```python
from build123d import *

# Parameters (mm, degrees)
SKETCH_2_R      = 3
SKETCH_2_R_2    = 1
EXTRUDE_1_DEPTH = 6
EXTRUDE_2_DEPTH = 5
SKETCH_6_R      = 3
SKETCH_6_R_2    = 1
EXTRUDE_3_DEPTH = 6
FILLET_1_R      = 1


with BuildPart() as part:
    # Эскиз2 → Бобышка-Вытянуть1 (new, symmetric)
    with BuildSketch(Plane.XY):
        Circle(SKETCH_2_R)
        Circle(SKETCH_2_R_2, mode=Mode.SUBTRACT)
    extrude(amount=EXTRUDE_1_DEPTH, both=True)

    # Эскиз4 → Бобышка-Вытянуть2 (add, symmetric)
    with BuildSketch(Plane.XY):
        with BuildLine():
            Line((2.236067977, 2), (23, 2))
            Line((23, 2), (23, -2))
            Line((23, -2), (2.236067977, -2))
            ThreePointArc((2.236067977, -2), (3, 0), (2.236067977, 2))
        make_face()
    extrude(amount=EXTRUDE_2_DEPTH, both=True)

    # Эскиз6 → Бобышка-Вытянуть3 (add, symmetric)
    with BuildSketch(Plane.XY):
        with Locations((24, 0)):
            Circle(SKETCH_6_R)
        with Locations((24, 0)):
            Circle(SKETCH_6_R_2, mode=Mode.SUBTRACT)
    extrude(amount=EXTRUDE_3_DEPTH, both=True)

    # Скругление1
    fillet_1_edges = [part.edges().sort_by_distance(p)[0] for p in [
        (2.802517077, 1.070466269, -5),
        (2.236067977, 2, 0),
        (2.236067977, -2, 0),
        (2.802517077, 1.070466269, 5),
        (21, 0, -5),
        (21.763932023, 2, 0),
        (21, 0, 5),
        (21.763932023, -2, 0),
    ]]
    fillet(fillet_1_edges, radius=FILLET_1_R - 0.0001)  # a hair under: the kernel refuses the full size


solid = part.part
```
Build history of the part. All positions in model axes, mm. A direction names the side the tool comes from. Round coordinates to 2 decimals unless told otherwise and drop trailing zeros. Order: outer loops, then holes, each group sorted by start corner. A loop starts at its lowest first (then second) coordinate and runs counter-clockwise, first axis right, second up. Notation, with made-up numbers: (-34.5, 73.25) - (-20.5, 73.25) arc R20 ccw to (-20.5, 94.25) - close; hole circle Ø2 at (56, 2.5). An arc over 180 degrees is marked (long way). Use a Markdown table: item, result.
1) Tool access for faces 4 (the face through (12, -2, 0)), 5 (the face through (12, 2, 0)), 6 (the face through (-3, 0, 0)): list every direction of +Z, -Z, +X, -X, +Y, -Y with a clear straight run to the whole face (end or side of a thin tool).
Recorded:
| item | result |
|---|---|
| face 4 | +Z, -Z, -Y |
| face 5 | +Z, -Z, +Y |
| face 6 | +Z, -Z |
2) Saw through at A-A on x = 0. Write the cut outline in (y, z), and give its area (3 significant figures).
Recorded:
| item | result |
|---|---|
| outline | (-3, -6) - (-1, -6) - (-1, 6) - (-3, 6) - close; (1, -6) - (3, -6) - (3, 6) - (1, 6) - close |
| area | 48.0 mm² |
3) Flat gauge pins, fed straight in: pin 1 Ø3 at (x, y) = (15.5, -1) entering from +Z; pin 2 Ø2 at (x, y) = (14, -1) entering from -Z; pin 3 Ø3 at (y, z) = (-2, 4.5) entering from -X. Where does each tip first touch, or does it go through?
Recorded:
| item | result |
|---|---|
| pin 1 | stops at z = 5 |
| pin 2 | stops at z = -5 |
| pin 3 | stops at x = -2.96 |
4) Saw through at D-D on y = 2.65. Write the cut outline in (x, z).
Recorded:
| item | result |
|---|---|
| outline | (-1.41, -6) - (1.41, -6) - (1.41, 6) - (-1.41, 6) - close; (22.59, -6) - (25.41, -6) - (25.41, 6) - (22.59, 6) - close |
5) Wall check: L1, parallel to X at y = -0.05, z = 4.5; L2, parallel to Y at x = 24, z = 3; L3, parallel to X at y = 0.9, z = 1. Give the ranges that are in metal, low to high.
Recorded:
| item | result |
|---|---|
| L1 | x = -3 to -1, 1 to 23, 25 to 27 |
| L2 | y = -3 to -1, 1 to 3 |
| L3 | x = -2.86 to -0.44, 0.44 to 23.56, 24.44 to 26.86 |
6) Pull direction Y, two halves, no side cores. Call faces 1 (the face through (0, -1, 0)), 2 (the face through (23, 1, 6)), 3 (the face through (26.77, -1.15, 0.08)): pulls with the +Y half, pulls with the -Y half, needs draft (parallel to the pull), parting line crosses it, or undercut.
Recorded:
| item | result |
|---|---|
| face 1 | undercut |
| face 2 | needs draft |
| face 3 | parting line crosses it |
7) Saw through at B-B on z = 3.75. Write the cut outline in (x, y), and give its area (3 significant figures).
Recorded:
| item | result |
|---|---|
| outline | (1.98, -2.25) arc R1 cw to (2.65, -2) - (21.35, -2) arc R1 cw to (22.02, -2.25) arc R3 ccw (long way) to (22.02, 2.25) arc R1 cw to (21.35, 2) - (2.65, 2) arc R1 cw to (1.98, 2.25) arc R3 ccw (long way) to start; hole circle Ø2 at (0, 0); hole circle Ø2 at (24, 0) |
| area | 124 mm² |
8) Saw through at C-C on y = 0. Give the number of separate pieces and of enclosed holes in the cut face, and give its area (3 significant figures).
Recorded:
| item | result |
|---|---|
| separate pieces | 3 |
| enclosed holes | 0 |
| area | 277 mm² |
